```python
from build123d import *

# Parameters (mm, degrees)
SKETCH1_R           = 62.5
BOSS_EXTRUDE1_DEPTH = 18
SKETCH2_R           = 27.5
CUT_EXTRUDE1_DEPTH  = 91.202549853
SKETCH3_R           = 3.859440813
CUT_EXTRUDE2_DEPTH  = 15.605006
CIRPATTERN1_START   = 2.394993892
CIRPATTERN1_DEPTH   = 15.605006108


# Read off the part's stored shape, not the designer's step: CirPattern1
with BuildPart() as part:
    # Sketch1 → Boss-Extrude1 (new body)
    with BuildSketch(Plane(origin=(0, 0, 0), x_dir=(1, 0, 0), z_dir=(0, 1, 0))):
        with Locations(Location((0, 0, 0), (0, 0, 270))):
            Circle(SKETCH1_R)
    extrude(amount=BOSS_EXTRUDE1_DEPTH)

    # Sketch2 → Cut-Extrude1 (cut, through all)
    with BuildSketch(Plane(origin=(0, 0, 0), x_dir=(1, 0, 0), z_dir=(0, 1, 0))):
        with Locations(Location((0, 0, 0), (0, 0, 270))):
            Circle(SKETCH2_R)
    extrude(amount=CUT_EXTRUDE1_DEPTH, mode=Mode.SUBTRACT)

    # Sketch3 → Cut-Extrude2 (cut)
    with BuildSketch(Plane(origin=(0, 18, 0), x_dir=(1, 0, 0), z_dir=(0, 1, 0))):
        with Locations((-25.929979996, 0)):
            Circle(SKETCH3_R)
    extrude(amount=-CUT_EXTRUDE2_DEPTH, mode=Mode.SUBTRACT)

    # CirPattern1 outline → CirPattern1 (cut)
    with BuildSketch(Plane(origin=(0, 0, 0), x_dir=(1, 0, 0), z_dir=(0, 1, 0)).offset(CIRPATTERN1_START)):
        with BuildLine():
            ThreePointArc((-10.492619379, -25.41957786), (-13.75, -23.815698604), (-16.76769049, -21.796663865))
            ThreePointArc((-16.76769049, -21.796663865), (-14.894710404, -25.798395185), (-10.492619379, -25.41957786))
        make_face()
        with BuildLine():
            ThreePointArc((-10.492619379, 25.41957786), (-14.894710404, 25.798395185), (-16.76769049, 21.796663865))
            ThreePointArc((-16.76769049, 21.796663865), (-13.75, 23.815698604), (-10.492619379, 25.41957786))
        make_face()
        with BuildLine():
            ThreePointArc((16.76769049, -21.796663865), (13.75, -23.815698604), (10.492619379, -25.41957786))
            ThreePointArc((10.492619379, -25.41957786), (14.894710404, -25.798395185), (16.76769049, -21.796663865))
        make_face()
        with BuildLine():
            ThreePointArc((16.76769049, 21.796663865), (14.894710404, 25.798395185), (10.492619379, 25.41957786))
            ThreePointArc((10.492619379, 25.41957786), (13.75, 23.815698604), (16.76769049, 21.796663865))
        make_face()
        with BuildLine():
            ThreePointArc((27.26030987, 3.622913995), (27.5, 0), (27.26030987, -3.622913995))
            ThreePointArc((27.26030987, -3.622913995), (29.789420809, 0), (27.26030987, 3.622913995))
        make_face()
    extrude(amount=CIRPATTERN1_DEPTH, mode=Mode.SUBTRACT)


solid = part.part
```
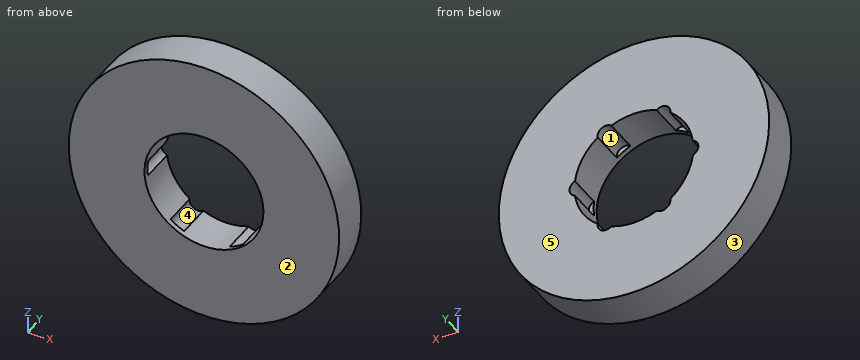
Check sheet for the modelled part. Datum: model origin and axes. Units: mm. Face numbers are marked on the shaded views. A direction names the side the tool comes from. Give positions to 0.01 mm unless a question says otherwise; leave off trailing zeros. Order: outer loops, then holes, each group sorted by start corner. A loop starts at its lowest first (then second) coordinate and runs counter-clockwise, first axis right, second up. Notation, with made-up numbers: (27.25, 69.25) -> (60.25, 69.25) arc R15 cw to (60.25, 90.25) -> close; hole circle Ø3 at (15.25, -8). An arc over 180 degrees is marked (long way). Return JSON: item names as keys, results as strings.
1. Set-up check for the marked faces 1 and 2: record each of +Z, -Z, +X, -X, +Y, -Y from which the full face is reachable in a straight line by a thin tool's end or side.
From the geometry:
{"face 1": "+Y", "face 2": "+Z, -Z, +X, -X, -Y"}
2. Go/stop test with flat-tipped pins: P1, Ø4, axis at x = -18, y = 8.5, coming from the +Z side; P2, Ø0.8, axis at x = -28.5, z = -0.5, coming from the +Y side (3 decimals); P3, Ø3, axis at y = 5, z = 16, coming from the +X side. Record where each tip stops, or that it passes through.
From the geometry:
{"P1": "z = 60.42", "P2": "y = 2.395", "P3": "x = 60.79"}
3. Cross-section at C-C, the plane y = 10. Record the cut outline in (x, z).
From the geometry:
{"outline": "circle Ø125 at (0, 0); hole (-27.26, -3.62) arc R27.5 ccw to (-16.77, -21.8) arc R3.86 ccw to (-10.49, -25.42) arc R27.5 ccw to (10.49, -25.42) arc R3.86 ccw to (16.77, -21.8) arc R27.5 ccw to (27.26, -3.62) arc R3.86 ccw to (27.26, 3.62) arc R27.5 ccw to (16.77, 21.8) arc R3.86 ccw to (10.49, 25.42) arc R27.5 ccw to (-10.49, 25.42) arc R3.86 ccw to (-16.77, 21.8) arc R27.5 ccw to (-27.26, 3.62) arc R3.86 ccw to start"}
4. Cross-section at A-A, the plane z = 0. Record the cut outline in (x, y) (3 decimals).
From the geometry:
{"outline": "(-62.5, 0) -> (-27.5, 0) -> (-27.5, 2.395) -> (-29.789, 2.395) -> (-29.789, 18) -> (-62.5, 18) -> close; (27.5, 0) -> (62.5, 0) -> (62.5, 18) -> (29.789, 18) -> (29.789, 2.395) -> (27.5, 2.395) -> close"}
5. Mould release check, pull along X, two halves, no side actions. Record for the marked faces 3, 4 and 5: +X half, -X half, draft (parallel to the pull), parting line (faces both ways), or undercut.
From the geometry:
{"face 3": "parting line", "face 4": "undercut", "face 5": "draft"}
6. Material ranges on probe 1 along Z at (x, y) = (1, 5.25); probe 2 along Z at (x, y) = (-25.5, 3); probe 3 along X at (y, z) = (3.25, -9.5), recorded low to high. Write a range as [from, to].
From the geometry:
{"probe 1": "[-62.49, -27.48], [27.48, 62.49]", "probe 2": "[-57.06, -10.3], [10.3, 57.06]", "probe 3": "[-61.77, -25.81], [25.81, 61.77]"}
7. Cross-section at B-B, the plane x = 0. Record the cut outline in (y, z).
From the geometry:
{"outline": "(0, -62.5) -> (18, -62.5) -> (18, -27.5) -> (0, -27.5) -> close; (0, 27.5) -> (18, 27.5) -> (18, 62.5) -> (0, 62.5) -> close"}
8. Cross-section at D-D, the plane x = -23.5. Record the cut outline in (y, z).
From the geometry:
{"outline": "(0, -57.91) -> (18, -57.91) -> (18, -14.28) -> (0, -14.28) -> close; (0, 14.28) -> (18, 14.28) -> (18, 57.91) -> (0, 57.91) -> close"}
